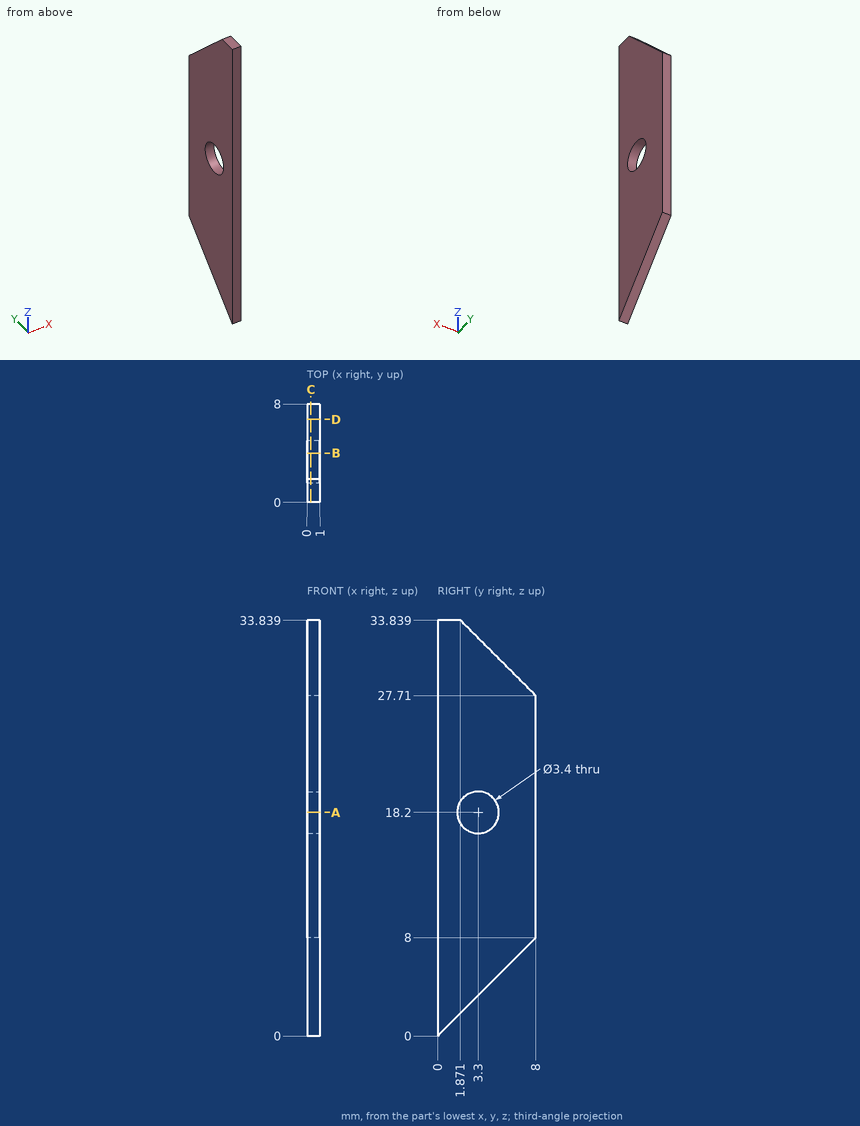
Geometry: see drawing. Coordinates: mm, zero at the bounding-box minimum. Give positions to 0.01 mm unless a question says otherwise; leave off trailing zeros. Write each loop counter-clockwise with the first axis right and the second up, starting at its lowest first coordinate (ties: lowest second). Pieces come first, ordered by that corner, then holes. Notation, with made-up numbers: M 79,55.25 L 99,55.25 A14 cw 99,73.25 Z; hole C 88,-32.75 d9. An arc over 180 degrees is marked long. Answer in a Markdown table with one row per item. Add a question column.
(1) Section D-D on y = 6.75. Return loops of the section in (x, z), and give its area (3 significant figures).
(2) Section A-A on z = 18.2. Return loops of the section in (x, y).
(3) Ray query, line 1 (Z direction, x = 0.45, y = 3.5); line 2 (Z direction, x = 0.65, y = 3.3); line 3 (Z direction, x = 0.95, y = 1.5). Return the intervals inside material, ascending.
(4) Section B-B on y = 4. Return loops of the section in (x, z).
(5) Section C-C on x = 0.3. Return loops of the section in (y, z), and give its area (3 significant figures).
Result set:
| question | item | result |
|---|---|---|
| 1 | outline | M 0,6.75 L 1,6.75 L 1,28.96 L 0,28.96 Z |
| 1 | area | 22.2 mm^2 |
| 2 | outline | M 0,0 L 1,0 L 1,1.6 L 0,1.6 Z; M 0,5 L 1,5 L 1,8 L 0,8 Z |
| 3 | line 1 | z = 3.5 to 16.51, 19.89 to 32.21 |
| 3 | line 2 | z = 3.3 to 16.5, 19.9 to 32.41 |
| 3 | line 3 | z = 1.5 to 33.84 |
| 4 | outline | M 0,4 L 1,4 L 1,16.65 L 0,16.65 Z; M 0,19.75 L 1,19.75 L 1,31.71 L 0,31.71 Z |
| 5 | outline | M 0,0 L 8,8 L 8,27.71 L 1.87,33.84 L 0,33.84 Z; hole C 3.3,18.2 d3.4 |
| 5 | area | 211 mm^2 |
